Check sheet for the modelled part. Datum: model origin and axes. Units: mm. Round coordinates to 2 decimals unless told otherwise and drop trailing zeros. Order: outer loops, then holes, each group sorted by start corner. A loop starts at its lowest first (then second) coordinate and runs counter-clockwise, first axis right, second up.
(1) Sectioned sample at D-D, the plane z = -31. Enter the section's corners in (x, y).
(2) Thickness scan on probe 1 along Z at (x, y) = (-10.75, 1); probe 2 along Z at (x, y) = (-10.75, 2.1); probe 3 along X at (y, z) = (1.35, -15.5). Record the ranges inside material, lowest first.
(3) Sectioned sample at B-B, the plane z = -11. Enter the section's corners in (x, y), and give its area (3 significant figures).
(4) Sectioned sample at C-C, the plane y = 2.2. Count the separate pieces of the cut face and the enclosed holes in it, and give its area (3 significant figures).
(5) Depth check by flat-ended pin: pin 1 (2 mm diameter, centred on x = -15, z = -28, fed in from +Y); pin 2 (2.5 mm diameter, centred on x = -18.75, z = -3, fed in from +Y); pin 3 (0.6 mm diameter, centred on x = -5, y = 3, fed in from +Z). Enter the tip coordinate at first touch or a pass-through.
(6) Sectioned sample at A-A, the plane x = -18.75. Enter the section's corners in (y, z).
Autodesk Inventor part; units mm, degrees
ref_plane "YZ Plane" through (0, 0, 0) normal (1, 0, 0) x (0, 1, 0)
ref_plane "XZ Plane" through (0, 0, 0) normal (0, 1, 0) x (-1, 0, 0)
ref_plane "XY Plane" through (0, 0, 0) normal (0, 0, 1) x (1, 0, 0)
sketch "Sketch1" plane through (0, 0, 0) normal (0, 1, 0) x (-1, 0, 0)
  line L0 (0, 0) -> (21.5, 0)
  line L1 (21.5, 0) -> (21.5, -51.5)
  line L2 (21.5, -51.5) -> (0, -51.5)
  line L3 (0, -51.5) -> (0, 0)
  line L4 (23.5, 2) -> (-2, 2)
  line L5 (-2, 2) -> (-2, -53.5)
  line L6 (-2, -53.5) -> (23.5, -53.5)
  line L7 (23.5, -53.5) -> (23.5, 2)
  line L8 (10.75, 0) -> (10.75, -51.5) construction
  circle A0 centre (10.75, -3) radius 1.5
  line L9 (0, -3) -> (21.5, -3) construction
  circle A1 centre (14.75, -3) radius 1.5
  circle A2 centre (18.75, -3) radius 1.5
  circle A3 centre (6.75, -3) radius 1.5
  circle A4 centre (2.75, -3) radius 1.5
  circle A5 centre (18.75, -7) radius 1.5
  circle A6 centre (14.75, -7) radius 1.5
  circle A7 centre (10.75, -7) radius 1.5
  circle A8 centre (6.75, -7) radius 1.5
  circle A9 centre (2.75, -7) radius 1.5
  circle A10 centre (18.75, -11) radius 1.5
  circle A11 centre (14.75, -11) radius 1.5
  circle A12 centre (10.75, -11) radius 1.5
  circle A13 centre (6.75, -11) radius 1.5
  circle A14 centre (2.75, -11) radius 1.5
  circle A15 centre (18.75, -15) radius 1.5
  circle A16 centre (14.75, -15) radius 1.5
  circle A17 centre (10.75, -15) radius 1.5
  circle A18 centre (6.75, -15) radius 1.5
  circle A19 centre (2.75, -15) radius 1.5
  point P0 (10.75, -3)
  point P1 (10.75, -7)
  point P2 (10.75, -11)
  point P3 (10.75, -15)
  dimension "d0" = 21.5
  dimension "d1" = 51.5
  dimension "d2" = 2
  dimension "d3" = 2
  dimension "d4" = 2
  dimension "d5" = 2
  dimension "d6" = 3
  dimension "d8" = 3
  dimension "d9" = 3
  dimension "d10" = 3
  dimension "d11" = 3
  dimension "d12" = 3
  dimension "d13" = 4
  dimension "d14" = 4
  dimension "d15" = 4
  dimension "d16" = 4
  dimension "d19" = 4
extrude "Extrusion1" add sketch "Sketch1" along normal blind 3 contours L0 L1 L2 L3 | L7 L6 L5 L4
fillet "Fillet1" radius 2 8 edges at (-23.5, 3, -25.75) (-10.75, 3, 2) (-23.5, 1.5, 2) (2, 1.5, 2) (2, 3, -25.75) (-10.75, 3, -53.5) (-23.5, 1.5, -53.5) (2, 1.5, -53.5)
sketch "Sketch2" plane through (0, 3, 0) normal (0, 1, 0) x (1, 0, 0)
  line L0 (-17.4247, 49.4836) -> (-8.1758, 49.4836) construction
  line L1 (-8.1758, 49.4836) -> (-8.1758, 43.1661) construction
  line L2 (-8.1758, 43.1661) -> (-17.4247, 43.1661) construction
  line L3 (-17.4247, 43.1661) -> (-17.4247, 49.4836) construction
  spline S0 degree 2 poles (-13.624, 39.0946) (-14.7099, 39.0946) (-16.2334, 39.5484) (-16.906, 39.8726) knots 0 0 0 1 2 2 2
  line L4 (-16.906, 39.8726) -> (-16.906, 41.5419)
  line L5 (-16.906, 41.5419) -> (-16.8088, 41.5419)
  spline S1 degree 2 poles (-16.8088, 41.5419) (-16.1524, 40.9261) (-14.4911, 40.2453) (-13.7213, 40.2453) knots 0 0 0 1 2 2 2
  spline S2 degree 2 poles (-13.7213, 40.2453) (-12.6192, 40.2453) (-11.4928, 41.1611) (-11.4928, 41.9147) knots 0 0 0 1 2 2 2
  spline S3 degree 2 poles (-11.4928, 41.9147) (-11.4928, 42.5144) (-12.0843, 43.2599) (-12.7245, 43.4463) knots 0 0 0 1 2 2 2
  spline S4 degree 2 poles (-12.7245, 43.4463) (-13.1864, 43.576) (-13.9563, 43.7543) (-14.5317, 43.9001) knots 0 0 0 1 2 2 2
  spline S5 degree 2 poles (-14.5317, 43.9001) (-15.0503, 44.0379) (-15.8688, 44.4512) (-16.1848, 44.7834) knots 0 0 0 1 2 2 2
  spline S6 degree 2 poles (-16.1848, 44.7834) (-16.4928, 45.1157) (-16.8331, 46.0071) (-16.8331, 46.5906) knots 0 0 0 1 2 2 2
  spline S7 degree 2 poles (-16.8331, 46.5906) (-16.8331, 47.8061) (-14.9368, 49.4512) (-13.4701, 49.4512) knots 0 0 0 1 2 2 2
  spline S8 degree 2 poles (-13.4701, 49.4512) (-12.6273, 49.4512) (-11.1362, 49.1189) (-10.496, 48.8029) knots 0 0 0 1 2 2 2
  line L6 (-10.496, 48.8029) -> (-10.496, 47.2146)
  line L7 (-10.496, 47.2146) -> (-10.5932, 47.2146)
  spline S9 degree 2 poles (-10.5932, 47.2146) (-11.0714, 47.6522) (-12.5624, 48.3005) (-13.3809, 48.3005) knots 0 0 0 1 2 2 2
  spline S10 degree 2 poles (-13.3809, 48.3005) (-14.3047, 48.3005) (-15.4474, 47.4334) (-15.4474, 46.7283) knots 0 0 0 1 2 2 2
  spline S11 degree 2 poles (-15.4474, 46.7283) (-15.4474, 46.0962) (-14.7748, 45.3426) (-14.1427, 45.1724) knots 0 0 0 1 2 2 2
  spline S12 degree 2 poles (-14.1427, 45.1724) (-13.7213, 45.059) (-12.4976, 44.7672) (-12.0924, 44.6457) knots 0 0 0 1 2 2 2
  spline S13 degree 2 poles (-12.0924, 44.6457) (-11.0633, 44.3296) (-10.107, 43.0573) (-10.107, 42.1254) knots 0 0 0 1 2 2 2
  spline S14 degree 2 poles (-10.107, 42.1254) (-10.107, 41.5338) (-10.5851, 40.3993) (-11.0146, 40.0022) knots 0 0 0 1 2 2 2
  spline S15 degree 2 poles (-11.0146, 40.0022) (-11.4928, 39.5646) (-12.7083, 39.0946) (-13.624, 39.0946) knots 0 0 0 1 2 2 2
  line L8 (-2.8704, 39.2729) -> (-9.0373, 39.2729)
  line L9 (-9.0373, 39.2729) -> (-9.0373, 40.691)
  spline S16 degree 2 poles (-9.0373, 40.691) (-8.3728, 41.315) (-7.1897, 42.4739) (-6.6224, 43.0979) knots 0 0 0 1 2 2 2
  spline S17 degree 2 poles (-6.6224, 43.0979) (-5.4798, 44.3539) (-4.6451, 45.8612) (-4.6451, 46.6635) knots 0 0 0 1 2 2 2
  spline S18 degree 2 poles (-4.6451, 46.6635) (-4.6451, 47.0849) (-4.9044, 47.717) (-5.1394, 47.9196) knots 0 0 0 1 2 2 2
  spline S19 degree 2 poles (-5.1394, 47.9196) (-5.3744, 48.1222) (-5.9903, 48.3248) (-6.3631, 48.3248) knots 0 0 0 1 2 2 2
  spline S20 degree 2 poles (-6.3631, 48.3248) (-6.7197, 48.3248) (-7.449, 48.1465) (-7.7812, 48.0087) knots 0 0 0 1 2 2 2
  spline S21 degree 2 poles (-7.7812, 48.0087) (-8.0649, 47.8953) (-8.5916, 47.5711) (-8.7537, 47.4577) knots 0 0 0 1 2 2 2
  line L10 (-8.7537, 47.4577) -> (-8.8266, 47.4577)
  line L11 (-8.8266, 47.4577) -> (-8.8266, 48.8839)
  spline S22 degree 2 poles (-8.8266, 48.8839) (-8.4133, 49.0865) (-6.9304, 49.4836) (-6.2659, 49.4836) knots 0 0 0 1 2 2 2
  spline S23 degree 2 poles (-6.2659, 49.4836) (-4.8639, 49.4836) (-3.2837, 48.0006) (-3.2837, 46.7364) knots 0 0 0 1 2 2 2
  spline S24 degree 2 poles (-3.2837, 46.7364) (-3.2837, 46.1449) (-3.5592, 45.1562) (-3.8023, 44.7348) knots 0 0 0 1 2 2 2
  spline S25 degree 2 poles (-3.8023, 44.7348) (-4.0454, 44.2972) (-4.7505, 43.4382) (-5.1394, 43.0249) knots 0 0 0 1 2 2 2
  spline S26 degree 2 poles (-5.1394, 43.0249) (-5.7715, 42.3361) (-7.3193, 40.8612) (-7.7812, 40.4317) knots 0 0 0 1 2 2 2
  line L12 (-7.7812, 40.4317) -> (-2.8704, 40.4317)
  line L13 (-2.8704, 40.4317) -> (-2.8704, 39.2729)
  point P0 (0, 0)
extrude "Extrusion2" add sketch "Sketch2" along normal blind 0.5
equation "\"d8\" = d6"
equation "\"d9\" = d11"
equation "\"d10\" = d11"
equation "\"d11\" = d6"
equation "\"d12\" = d11"
equation "\"d14\" = d13"
equation "\"d16\" = d15"
properties part number "sensor2"
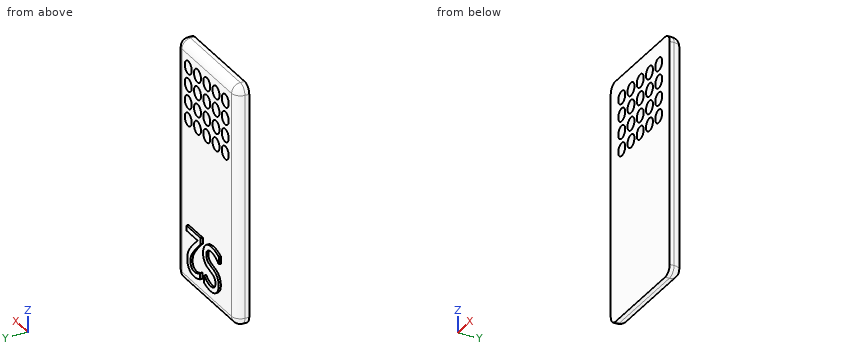
Derived:
1. outline: (-23.5, 0) - (2, 0) - (2, 1) arc R2 ccw to (0, 3) - (-21.5, 3) arc R2 ccw to (-23.5, 1) - close
2. probe 1: z = -53.5 to -16.5, -13.5 to -12.5, -9.5 to -8.5, -5.5 to -4.5, -1.5 to 2
2. probe 2: z = -53.17 to -16.5, -13.5 to -12.5, -9.5 to -8.5, -5.5 to -4.5, -1.5 to 1.67
2. probe 3: x = -23.47 to -20.16, -17.34 to -16.16, -13.34 to -12.16, -9.34 to -8.16, -5.34 to -4.16, -1.34 to 1.97
3. outline: (-23.5, 0) - (-20.25, 0) - (-20.25, 3) - (-21.5, 3) arc R2 ccw to (-23.5, 1) - close; (-17.25, 0) - (-16.25, 0) - (-16.25, 3) - (-17.25, 3) - close; (-13.25, 0) - (-12.25, 0) - (-12.25, 3) - (-13.25, 3) - close; (-9.25, 0) - (-8.25, 0) - (-8.25, 3) - (-9.25, 3) - close; (-5.25, 0) - (-4.25, 0) - (-4.25, 3) - (-5.25, 3) - close; (-1.25, 0) - (2, 0) - (2, 1) arc R2 ccw to (0, 3) - (-1.25, 3) - close
3. area: 29.8 mm2
4. separate pieces: 1
4. enclosed holes: 20
4. area: 1,210 mm2
5. pin 1: stops at y = 3
5. pin 2: passes through
5. pin 3: stops at z = 1.05
6. outline: (0, -53.5) - (1, -53.5) arc R2 ccw to (3, -51.5) - (3, -16.5) - (0, -16.5) - close; (0, -13.5) - (3, -13.5) - (3, -12.5) - (0, -12.5) - close; (0, -9.5) - (3, -9.5) - (3, -8.5) - (0, -8.5) - close; (0, -5.5) - (3, -5.5) - (3, -4.5) - (0, -4.5) - close; (0, -1.5) - (3, -1.5) - (3, 0) arc R2 ccw to (1, 2) - (0, 2) - close
